Check sheet for the modelled part. Datum: model origin and axes. Units: mm. Give positions to 0.01 mm unless a question says otherwise; leave off trailing zeros. Order: outer loops, then holes, each group sorted by start corner. A loop starts at its lowest first (then second) coordinate and runs counter-clockwise, first axis right, second up. Notation, with made-up numbers: (45.25, -14.75) -> (102.25, -14.75) arc R16 cw to (102.25, 0.25) -> close; hole circle Ø9 at (-26.75, 51). An arc over 180 degrees is marked (long way). Answer in a Markdown table with one row per item. Add a question column.
(1) Cross-section at A-A (y = 2). Record the cut outline in (x, z).
(2) Thickness scan on L1, parallel to Y at x = 13.5, z = -0.75; L2, parallel to Y at x = 0.5, z = -0.05; L3, parallel to X at y = -13.5, z = -0.9. Record the ranges inside material, lowest first. Write a range as [from, to].
(3) Cross-section at D-D (z = -1.15). State how many separate pieces and enclosed holes the cut face has, then the cut area to 3 significant figures.
(4) Go/stop test with a flat-tipped pin: pin 1 (1 mm diameter, centred on y = 6, z = -0.5, fed in from +X). Record where the tip stops, or that it passes through.
(5) Cross-section at C-C (y = -12.5). Record the cut outline in (x, z).
(6) Cross-section at B-B (x = -4). Record the cut outline in (y, z), then the cut area to 3 significant figures.
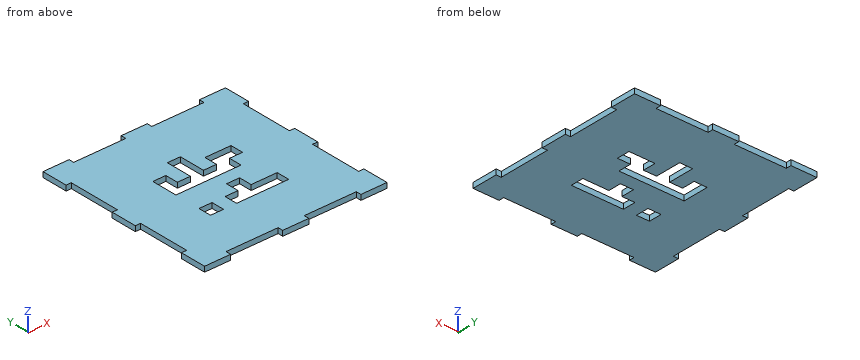
```python
from build123d import *

# Parameters (mm, degrees)
SKETCH1_W           = 70
SKETCH1_H           = 70
BOSS_EXTRUDE1_DEPTH = 2
SKETCH2_W           = 2
SKETCH2_H           = 20
SKETCH2_W_2         = 20
SKETCH2_H_2         = 2
CUT_EXTRUDE1_DEPTH  = 2
SKETCH3_W           = 5
SKETCH3_H           = 5
CUT_EXTRUDE5_DEPTH  = 10


with BuildPart() as part:
    # Sketch1 → Boss-Extrude1 (new body)
    with BuildSketch(Plane.XY):
        Rectangle(SKETCH1_W, SKETCH1_H)
    extrude(amount=-BOSS_EXTRUDE1_DEPTH)

    # Sketch2 → Cut-Extrude1 (cut)
    with BuildSketch(Plane.XY):
        with Locations((-34, 15)):
            Rectangle(SKETCH2_W, SKETCH2_H)
        with Locations((-34, -15)):
            Rectangle(SKETCH2_W, SKETCH2_H)
        with Locations((-15, -34)):
            Rectangle(SKETCH2_W_2, SKETCH2_H_2)
        with Locations((15, -34)):
            Rectangle(SKETCH2_W_2, SKETCH2_H_2)
        with Locations((34, -15)):
            Rectangle(SKETCH2_W, SKETCH2_H)
        with Locations((34, 15)):
            Rectangle(SKETCH2_W, SKETCH2_H)
        with Locations((15, 34)):
            Rectangle(SKETCH2_W_2, SKETCH2_H_2)
        with Locations((-15, 34)):
            Rectangle(SKETCH2_W_2, SKETCH2_H_2)
    extrude(amount=-CUT_EXTRUDE1_DEPTH, mode=Mode.SUBTRACT)

    # Sketch3 → Cut-Extrude5 (cut)
    with BuildSketch(Plane.XY):
        with Locations((-12.5, 7.5)):
            Rectangle(SKETCH3_W, SKETCH3_H)
        with Locations((-12.5, 2.5)):
            Rectangle(SKETCH3_W, SKETCH3_H)
        with Locations((-7.5, 2.5)):
            Rectangle(SKETCH3_W, SKETCH3_H)
        with Locations((-2.5, 2.5)):
            Rectangle(SKETCH3_W, SKETCH3_H)
        with Locations((2.5, 2.5)):
            Rectangle(SKETCH3_W, SKETCH3_H)
        with Locations((7.5, 2.5)):
            Rectangle(SKETCH3_W, SKETCH3_H)
        with Locations((7.5, 7.5)):
            Rectangle(SKETCH3_W, SKETCH3_H)
        with Locations((12.5, 7.5)):
            Rectangle(SKETCH3_W, SKETCH3_H)
        with Locations((-2.5, 7.5)):
            Rectangle(SKETCH3_W, SKETCH3_H)
        with Locations((-2.5, 12.5)):
            Rectangle(SKETCH3_W, SKETCH3_H)
        with Locations((-12.5, -12.5)):
            Rectangle(SKETCH3_W, SKETCH3_H)
        with Locations((-2.5, -12.5)):
            Rectangle(SKETCH3_W, SKETCH3_H)
        with Locations((2.5, -12.5)):
            Rectangle(SKETCH3_W, SKETCH3_H)
        with Locations((7.5, -12.5)):
            Rectangle(SKETCH3_W, SKETCH3_H)
        with Locations((12.5, -12.5)):
            Rectangle(SKETCH3_W, SKETCH3_H)
        with Locations((2.5, -7.5)):
            Rectangle(SKETCH3_W, SKETCH3_H)
    extrude(amount=-CUT_EXTRUDE5_DEPTH, mode=Mode.SUBTRACT)


solid = part.part
```
Answer below:
| question | item | result |
|---|---|---|
| 1 | outline | (-35, -2) -> (-15, -2) -> (-15, 0) -> (-35, 0) -> close; (10, -2) -> (35, -2) -> (35, 0) -> (10, 0) -> close |
| 2 | L1 | y = [-33, -15], [-10, 5], [10, 33] |
| 2 | L2 | y = [-35, -15], [-5, 0], [5, 35] |
| 2 | L3 | x = [-33, -15], [-10, -5], [15, 33] |
| 3 | separate pieces | 1 |
| 3 | enclosed holes | 3 |
| 3 | area | 4,180 mm² |
| 4 | pin 1 | stops at x = 33 |
| 5 | outline | (-33, -2) -> (-15, -2) -> (-15, 0) -> (-33, 0) -> close; (-10, -2) -> (-5, -2) -> (-5, 0) -> (-10, 0) -> close; (15, -2) -> (33, -2) -> (33, 0) -> (15, 0) -> close |
| 6 | outline | (-35, -2) -> (-15, -2) -> (-15, 0) -> (-35, 0) -> close; (-10, -2) -> (0, -2) -> (0, 0) -> (-10, 0) -> close; (15, -2) -> (35, -2) -> (35, 0) -> (15, 0) -> close |
| 6 | area | 100 mm² |
